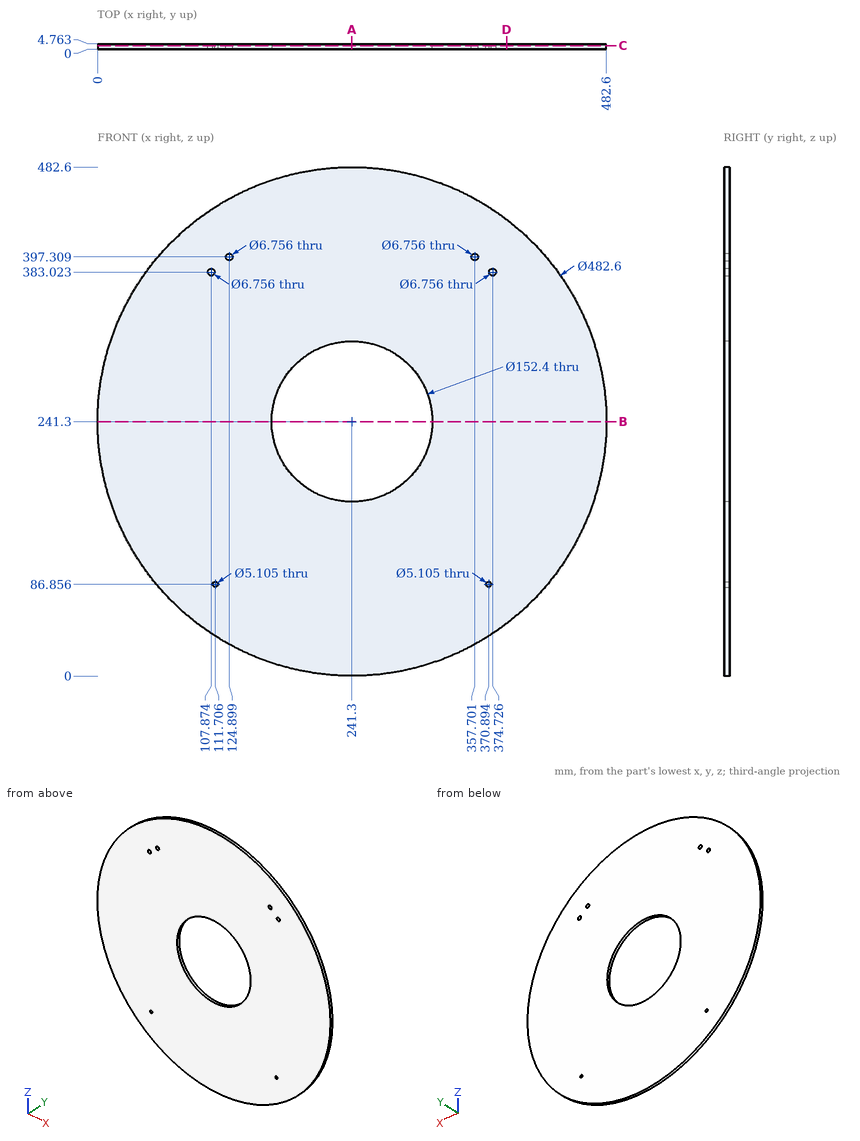
Geometry: see drawing. Coordinates: mm, zero at the bounding-box minimum. Round coordinates to 2 decimals unless told otherwise and drop trailing zeros. Write each loop counter-clockwise with the first axis right and the second up, starting at its lowest first coordinate (ties: lowest second). Pieces come first, ordered by that corner, then holes. Notation, with made-up numbers: (-25.75, 86.25) - (3.25, 86.25) arc R25 ccw to (3.25, 116.25) - close; hole circle Ø7 at (81, -29). An arc over 180 degrees is marked (long way). Use CSV: the item, a comma, the result in double quotes. Start each with the question number.
(1) Cut plane A-A, the plane x = 241.3. Return loops of the section in (y, z), and give its area (3 significant figures).
(2) Cut plane D-D, the plane x = 388. Return loops of the section in (y, z) (1 decimal).
(3) First-contact query: pin 1 Ø11 at (x, z) = (357.7, 397.31) entering from -Y; pin 2 Ø1.5 at (y, z) = (2.5, 374) entering from -X. Flat tips, straight axial feed; report the tip coordinate or a pass-through.
(4) Cut plane B-B, the plane z = 241.3. Return loops of the section in (x, y), and give its area (3 significant figures).
(5) Material intervals for probe 1 along X at (y, z) = (2.75, 241); probe 2 along Z at (x, y) = (446.5, 2.2) (1 decimal); probe 3 along Z at (x, y) = (42.5, 4.2) (1 decimal), sorted ascending. Write a range as [from, to].
(6) Cut plane C-C, the plane y = 3.1. Return loops of the section in (x, z) (1 decimal), and give its area (3 significant figures).
Geometry says:
1,outline,"(0, 0) - (4.76, 0) - (4.76, 165.1) - (0, 165.1) - close; (0, 317.5) - (4.76, 317.5) - (4.76, 482.6) - (0, 482.6) - close"
1,area,"1,570 mm²"
2,outline,"(0, 49.7) - (4.8, 49.7) - (4.8, 432.9) - (0, 432.9) - close"
3,pin 1,"y = 0"
3,pin 2,"x = 39.27"
4,outline,"(0, 0) - (165.1, 0) - (165.1, 4.76) - (0, 4.76) - close; (317.5, 0) - (482.6, 0) - (482.6, 4.76) - (317.5, 4.76) - close"
4,area,"1,570 mm²"
5,probe 1,"[0, 165.1], [317.5, 482.6]"
5,probe 2,"[114.3, 368.3]"
5,probe 3,"[104.5, 378.1]"
6,outline,"circle Ø482.6 at (241.3, 241.3); hole circle Ø6.8 at (107.9, 383); hole circle Ø5.1 at (111.7, 86.9); hole circle Ø6.8 at (124.9, 397.3); hole circle Ø152.4 at (241.3, 241.3); hole circle Ø6.8 at (357.7, 397.3); hole circle Ø5.1 at (370.9, 86.9); hole circle Ø6.8 at (374.7, 383)"
6,area,"164,000 mm²"
